Build history of the part. All positions in model axes, mm. Face numbers are marked on the shaded views. A direction names the side the tool comes from. Round coordinates to 2 decimals unless told otherwise and drop trailing zeros. Loops run counter-clockwise (first coordinate to the right, second up) from the corner with the lowest first, then second, coordinate; pieces in that order, holes last. Notation, with made-up numbers: (57.5, -17.75) - (64.5, -17.75) arc R26 cw to (64.5, 17.25) - close; hole circle Ø10 at (45.5, -11.5). An arc over 180 degrees is marked (long way). Use a Markdown table: item, result.
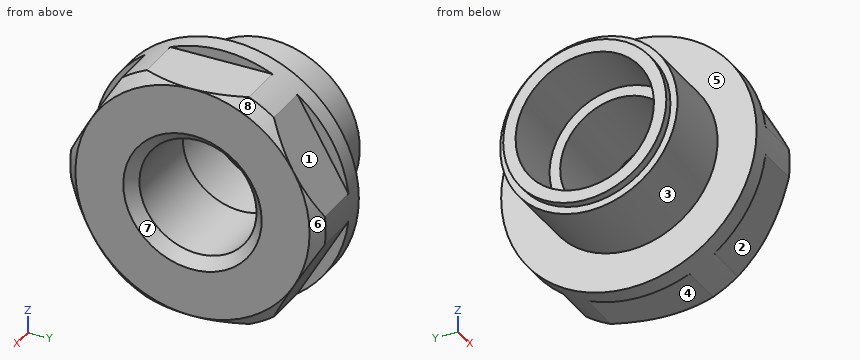
from build123d import *

# Parameters (mm, degrees)
TAGLIO_ESTRUSIONE1_DEPTH      = 5.25
TAGLIO_ESTRUSIONE1_DEPTH_BACK = 5.25
TAGLIO_ESTRUSIONE2_DEPTH      = 5.25
TAGLIO_ESTRUSIONE2_DEPTH_BACK = 5.25


with BuildPart() as part:
    # Schizzo1 → Rivoluzione1 (revolve)
    with BuildSketch(Plane.XY, mode=Mode.PRIVATE) as rivoluzione1_sk:
        Polygon((0, 6.5), (6.153846154, 6.5), (6.153846154, 5.5), (14, 5.5), (15, 6.5), (15, 11), (14, 12), (8, 12), (8, 8.33), (0.740444444, 8.33), (0.740444444, 7.6636), (0, 7.6636), align=None)
    revolve(rivoluzione1_sk.sketch.rotate(Axis((15, 0, 0), (-1, 0, 0)), 270), axis=Axis((15, 0, 0), (-1, 0, 0)))

    # Schizzo2 → Taglio-Estrusione1 (cut, two sides: drawn at the far end of the back side and taken through both)
    with BuildSketch(Plane(origin=(15, 0, 0), x_dir=(0, 0, -1), z_dir=(1, 0, 0)).offset(-TAGLIO_ESTRUSIONE1_DEPTH_BACK)):
        Polygon((-16.5, -9.526279442), (1, -19.629909152), (1, -13.279056191), (-11, -6.350852961), (-11, 6.350852961), (1, 13.279056191), (1, 19.629909152), (-16.5, 9.526279442), align=None)
    extrude(amount=TAGLIO_ESTRUSIONE1_DEPTH + TAGLIO_ESTRUSIONE1_DEPTH_BACK, mode=Mode.SUBTRACT)

    # Schizzo3 → Taglio-Estrusione2 (cut, two sides: drawn at the far end of the back side and taken through both)
    with BuildSketch(Plane(origin=(15, 0, 0), x_dir=(0, 0, -1), z_dir=(1, 0, 0)).offset(-TAGLIO_ESTRUSIONE2_DEPTH_BACK)):
        Polygon((-1, -19.629909152), (16.5, -9.526279442), (16.5, 9.526279442), (-1, 19.629909152), (-1, 13.279056191), (11, 6.350852961), (11, -6.350852961), (-1, -13.279056191), align=None)
    extrude(amount=TAGLIO_ESTRUSIONE2_DEPTH + TAGLIO_ESTRUSIONE2_DEPTH_BACK, mode=Mode.SUBTRACT)


solid = part.part
Q1. Cut at A-A, the plane x = 11.75. List the corners of the cut face in (y, z).
Results found:
| item | result |
|---|---|
| outline | (-11.92, -1.35) - (-7.13, -9.65) arc R12 ccw to (-4.8, -11) - (4.8, -11) arc R12 ccw to (7.13, -9.65) - (11.92, -1.35) arc R12 ccw to (11.92, 1.35) - (7.13, 9.65) arc R12 ccw to (4.8, 11) - (-4.8, 11) arc R12 ccw to (-7.13, 9.65) - (-11.92, 1.35) arc R12 ccw to start; hole circle Ø11 at (0, 0) |
Q2. Drop flat-ended pins along their axis: pin 1 (1.5 mm diameter, centred on x = 9.5, z = -2.5, fed in from +Y); pin 2 (8 mm diameter, centred on x = 3.5, y = -7.5, fed in from -Z); pin 3 (8 mm diameter, centred on x = 2, z = -8, fed in from -Y). Give the stop position or say it passes through.
Results found:
| item | result |
|---|---|
| pin 1 | stops at y = 11.87 |
| pin 2 | stops at z = -7.56 |
| pin 3 | stops at y = -7.31 |
Q3. Cut at C-C, the plane x = 7.25. List the corners of the cut face in (y, z).
Results found:
| item | result |
|---|---|
| outline | circle Ø16.66 at (0, 0); hole circle Ø11 at (0, 0) |
Q4. Cut at B-B, the plane z = 0. List the corners of the cut face in (x, y), plus the area to 3 significant figures.
Results found:
| item | result |
|---|---|
| outline | (0, -7.66) - (0.74, -7.66) - (0.74, -8.33) - (8, -8.33) - (8, -12) - (14, -12) - (15, -11) - (15, -6.5) - (14, -5.5) - (6.15, -5.5) - (6.15, -6.5) - (0, -6.5) - close; (0, 6.5) - (6.15, 6.5) - (6.15, 5.5) - (14, 5.5) - (15, 6.5) - (15, 11) - (14, 12) - (8, 12) - (8, 8.33) - (0.74, 8.33) - (0.74, 7.66) - (0, 7.66) - close |
| area | 121 mm2 |
Q5. Which spindle directions (+Z, -Z, +X, -X, +Y, -Y) get a long thin tool onto all of the face, cutting with end or side? Do the marked faces 1, 2, 3 and 4. Say none if no direction does.
Results found:
| item | result |
|---|---|
| face 1 | +Z, +X, +Y |
| face 2 | -Z, +X, -Y |
| face 3 | -X |
| face 4 | -Z, +X, +Y, -Y |
Q6. Pull direction Z, two halves, no side cores. Call the marked faces 5, 6, 7 and 8: pulls with the +Z half, pulls with the -Z half, needs draft (parallel to the pull), parting line crosses it, or undercut.
Results found:
| item | result |
|---|---|
| face 5 | needs draft |
| face 6 | parting line crosses it |
| face 7 | undercut |
| face 8 | pulls with the +Z half |
Q7. Probe line 1 (Y direction, x = 10.25, z = 0); line 2 (Y direction, x = 2.75, z = 0); line 3 (X direction, y = 8.75, z = -6.25). List the from-to ranges inside material, lowest first.
Results found:
| item | result |
|---|---|
| line 1 | y = -12 to -5.5, 5.5 to 12 |
| line 2 | y = -8.33 to -6.5, 6.5 to 8.33 |
| line 3 | x = 8 to 15 |
